Check sheet for the modelled part. Datum: model origin and axes. Units: mm. Face numbers are marked on the shaded views. A direction names the side the tool comes from. Give positions to 0.01 mm unless a question says otherwise; leave off trailing zeros. Order: outer loops, then holes, each group sorted by start corner. A loop starts at its lowest first (then second) coordinate and runs counter-clockwise, first axis right, second up.
Item 1: Sectioned sample at A-A on x = 0. Record the boundary of the cut face in (y, z), and give its area (3 significant figures).
Item 2: Sectioned sample at B-B on z = 0.7. Record the boundary of the cut face in (x, y) (3 decimals), and give its area (3 significant figures).
Item 3: Access from +Z, -Z, +X, -X, +Y, -Y to the whole of each face (thin tool, end or side, straight path). Record for the marked faces 1, 2 and 3.
Item 4: Release check for a two-part mould opening along X. For the marked faces 4, 5, 6 and 7 record: released by +X, released by -X, zero draft, split by the parting line, or undercut.
Item 5: Material ranges on line 1 along X through (y, z) = (-1, 2.4); line 2 along Y through (x, z) = (0, 0.75); line 3 along Z through (x, y) = (6.5, -9.5), recorded low to high.
Item 6: Gauge pin test, flat ends, axial feed: P1, Ø3.5, axis at x = -6.5, y = -9.5, coming from the +Z side; P2, Ø0.6, axis at x = -2.5, y = 5.5, coming from the +Z side; P3, Ø0.8, axis at x = -11.5, y = -0.5, coming from the +Z side. Record the tip position at first contact, or that the pin passes through.
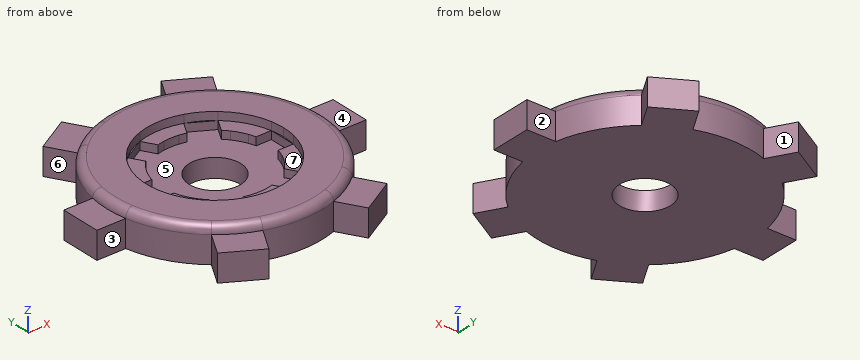
from build123d import *

# Parameters (mm, degrees)
F2_DEPTH = 2.54
F3_R     = 7.6884407039
F3_R_2   = 2.4226171542
F4_DEPTH = 1.778
F6_DEPTH = 0.762
F7_R     = 0.76199


# Not quite as in the source:
# - a fillet or chamfer is up to 0.001 mm smaller than in the source, because OpenCascade refuses the exact size


with BuildPart() as f2:
    # F1 (on Top) → F2 (new body)
    with BuildSketch(Plane.XY):
        with BuildLine():
            ThreePointArc((9.9798083649, -1.905), (10.1148517781, -0.9567515385), (10.16, 0))
            ThreePointArc((10.16, 0), (10.1148517781, 0.9567515385), (9.9798083649, 1.905))
            Line((9.9798083649, 1.905), (4.7092860393, 1.905))
            ThreePointArc((4.7092860393, 1.905), (4.8244462237, 1.5909489729), (4.9186888497, 1.27))
            Line((4.9186888497, 1.27), (6.35, 1.27))
            Line((6.35, 1.27), (6.35, -1.27))
            Line((6.35, -1.27), (4.9186888497, -1.27))
            ThreePointArc((4.9186888497, -1.27), (4.8244462237, -1.5909489729), (4.7092860393, -1.905))
            Line((4.7092860393, -1.905), (9.9798083649, -1.905))
        make_face()
        with BuildLine():
            ThreePointArc((9.9798083649, 1.905), (10.1148517781, 0.9567515385), (10.16, 0))
            ThreePointArc((10.16, 0), (10.1148517781, -0.9567515385), (9.9798083649, -1.905))
            Line((9.9798083649, -1.905), (12.7, -1.905))
            Line((12.7, -1.905), (12.7, 1.905))
            Line((12.7, 1.905), (9.9798083649, 1.905))
        make_face()
        with BuildLine():
            Line((4.7092860393, 1.905), (9.9798083649, 1.905))
            ThreePointArc((9.9798083649, 1.905), (8.7988181024, 5.08), (6.6396825767, 7.6902675689))
            Line((6.6396825767, 7.6902675689), (4.0044214139, 3.1258613437))
            ThreePointArc((4.0044214139, 3.1258613437), (4.3994090512, 2.54), (4.7092860393, 1.905))
        make_face()
        with BuildLine():
            ThreePointArc((6.6396825767, -7.6902675689), (8.7988181024, -5.08), (9.9798083649, -1.905))
            Line((9.9798083649, -1.905), (4.7092860393, -1.905))
            ThreePointArc((4.7092860393, -1.905), (4.3994090512, -2.54), (4.0044214139, -3.1258613437))
            Line((4.0044214139, -3.1258613437), (6.6396825767, -7.6902675689))
        make_face()
        with BuildLine():
            Line((4.0044214139, 3.1258613437), (6.6396825767, 7.6902675689))
            ThreePointArc((6.6396825767, 7.6902675689), (5.08, 8.7988181024), (3.3401257882, 9.5952675689))
            Line((3.3401257882, 9.5952675689), (0.7048646254, 5.0308613437))
            ThreePointArc((0.7048646254, 5.0308613437), (1.0344208852, 4.9735674754), (1.359492162, 4.8947094971))
            Line((1.359492162, 4.8947094971), (2.0751477372, 6.134261314))
            Line((2.0751477372, 6.134261314), (4.2748522628, 4.864261314))
            Line((4.2748522628, 4.864261314), (3.5591966876, 3.6247094971))
            ThreePointArc((3.5591966876, 3.6247094971), (3.7900253385, 3.3826185025), (4.0044214139, 3.1258613437))
        make_face()
        with BuildLine():
            ThreePointArc((3.3401257882, 9.5952675689), (5.08, 8.7988181024), (6.6396825767, 7.6902675689))
            Line((6.6396825767, 7.6902675689), (7.9997783942, 10.0460226281))
            Line((7.9997783942, 10.0460226281), (4.7002216058, 11.9510226281))
            Line((4.7002216058, 11.9510226281), (3.3401257882, 9.5952675689))
        make_face()
        with BuildLine():
            Line((7.9997783942, -10.0460226281), (6.6396825767, -7.6902675689))
            ThreePointArc((6.6396825767, -7.6902675689), (5.08, -8.7988181024), (3.3401257882, -9.5952675689))
            Line((3.3401257882, -9.5952675689), (4.7002216058, -11.9510226281))
            Line((4.7002216058, -11.9510226281), (7.9997783942, -10.0460226281))
        make_face()
        with BuildLine():
            ThreePointArc((3.3401257882, -9.5952675689), (5.08, -8.7988181024), (6.6396825767, -7.6902675689))
            Line((6.6396825767, -7.6902675689), (4.0044214139, -3.1258613437))
            ThreePointArc((4.0044214139, -3.1258613437), (3.7900253385, -3.3826185025), (3.5591966876, -3.6247094971))
            Line((3.5591966876, -3.6247094971), (4.2748522628, -4.864261314))
            Line((4.2748522628, -4.864261314), (2.0751477372, -6.134261314))
            Line((2.0751477372, -6.134261314), (1.359492162, -4.8947094971))
            ThreePointArc((1.359492162, -4.8947094971), (1.0344208852, -4.9735674754), (0.7048646254, -5.0308613437))
            Line((0.7048646254, -5.0308613437), (3.3401257882, -9.5952675689))
        make_face()
        with BuildLine():
            Line((0.7048646254, 5.0308613437), (3.3401257882, 9.5952675689))
            ThreePointArc((3.3401257882, 9.5952675689), (0, 10.16), (-3.3401257882, 9.5952675689))
            Line((-3.3401257882, 9.5952675689), (-0.7048646254, 5.0308613437))
            ThreePointArc((-0.7048646254, 5.0308613437), (0, 5.08), (0.7048646254, 5.0308613437))
        make_face()
        with BuildLine():
            ThreePointArc((-3.3401257882, -9.5952675689), (0, -10.16), (3.3401257882, -9.5952675689))
            Line((3.3401257882, -9.5952675689), (0.7048646254, -5.0308613437))
            ThreePointArc((0.7048646254, -5.0308613437), (0, -5.08), (-0.7048646254, -5.0308613437))
            Line((-0.7048646254, -5.0308613437), (-3.3401257882, -9.5952675689))
        make_face()
        with BuildLine():
            Line((-0.7048646254, 5.0308613437), (-3.3401257882, 9.5952675689))
            ThreePointArc((-3.3401257882, 9.5952675689), (-5.08, 8.7988181024), (-6.6396825767, 7.6902675689))
            Line((-6.6396825767, 7.6902675689), (-4.0044214139, 3.1258613437))
            ThreePointArc((-4.0044214139, 3.1258613437), (-3.7900253385, 3.3826185025), (-3.5591966876, 3.6247094971))
            Line((-3.5591966876, 3.6247094971), (-4.2748522628, 4.864261314))
            Line((-4.2748522628, 4.864261314), (-2.0751477372, 6.134261314))
            Line((-2.0751477372, 6.134261314), (-1.359492162, 4.8947094971))
            ThreePointArc((-1.359492162, 4.8947094971), (-1.0344208852, 4.9735674754), (-0.7048646254, 5.0308613437))
        make_face()
        with BuildLine():
            ThreePointArc((-6.6396825767, 7.6902675689), (-5.08, 8.7988181024), (-3.3401257882, 9.5952675689))
            Line((-3.3401257882, 9.5952675689), (-4.7002216058, 11.9510226281))
            Line((-4.7002216058, 11.9510226281), (-7.9997783942, 10.0460226281))
            Line((-7.9997783942, 10.0460226281), (-6.6396825767, 7.6902675689))
        make_face()
        with BuildLine():
            Line((-4.7002216058, -11.9510226281), (-3.3401257882, -9.5952675689))
            ThreePointArc((-3.3401257882, -9.5952675689), (-5.08, -8.7988181024), (-6.6396825767, -7.6902675689))
            Line((-6.6396825767, -7.6902675689), (-7.9997783942, -10.0460226281))
            Line((-7.9997783942, -10.0460226281), (-4.7002216058, -11.9510226281))
        make_face()
        with BuildLine():
            ThreePointArc((-6.6396825767, -7.6902675689), (-5.08, -8.7988181024), (-3.3401257882, -9.5952675689))
            Line((-3.3401257882, -9.5952675689), (-0.7048646254, -5.0308613437))
            ThreePointArc((-0.7048646254, -5.0308613437), (-1.0344208852, -4.9735674754), (-1.359492162, -4.8947094971))
            Line((-1.359492162, -4.8947094971), (-2.0751477372, -6.134261314))
            Line((-2.0751477372, -6.134261314), (-4.2748522628, -4.864261314))
            Line((-4.2748522628, -4.864261314), (-3.5591966876, -3.6247094971))
            ThreePointArc((-3.5591966876, -3.6247094971), (-3.7900253385, -3.3826185025), (-4.0044214139, -3.1258613437))
            Line((-4.0044214139, -3.1258613437), (-6.6396825767, -7.6902675689))
        make_face()
        with BuildLine():
            Line((-4.0044214139, 3.1258613437), (-6.6396825767, 7.6902675689))
            ThreePointArc((-6.6396825767, 7.6902675689), (-8.7988181024, 5.08), (-9.9798083649, 1.905))
            Line((-9.9798083649, 1.905), (-4.7092860393, 1.905))
            ThreePointArc((-4.7092860393, 1.905), (-4.3994090512, 2.54), (-4.0044214139, 3.1258613437))
        make_face()
        with BuildLine():
            ThreePointArc((-9.9798083649, -1.905), (-8.7988181024, -5.08), (-6.6396825767, -7.6902675689))
            Line((-6.6396825767, -7.6902675689), (-4.0044214139, -3.1258613437))
            ThreePointArc((-4.0044214139, -3.1258613437), (-4.3994090512, -2.54), (-4.7092860393, -1.905))
            Line((-4.7092860393, -1.905), (-9.9798083649, -1.905))
        make_face()
        with BuildLine():
            Line((-4.7092860393, 1.905), (-9.9798083649, 1.905))
            ThreePointArc((-9.9798083649, 1.905), (-10.16, 0), (-9.9798083649, -1.905))
            Line((-9.9798083649, -1.905), (-4.7092860393, -1.905))
            ThreePointArc((-4.7092860393, -1.905), (-4.8244462237, -1.5909489729), (-4.9186888497, -1.27))
            Line((-4.9186888497, -1.27), (-6.35, -1.27))
            Line((-6.35, -1.27), (-6.35, 1.27))
            Line((-6.35, 1.27), (-4.9186888497, 1.27))
            ThreePointArc((-4.9186888497, 1.27), (-4.8244462237, 1.5909489729), (-4.7092860393, 1.905))
        make_face()
        with BuildLine():
            ThreePointArc((-9.9798083649, -1.905), (-10.16, 0), (-9.9798083649, 1.905))
            Line((-9.9798083649, 1.905), (-12.7, 1.905))
            Line((-12.7, 1.905), (-12.7, -1.905))
            Line((-12.7, -1.905), (-9.9798083649, -1.905))
        make_face()
    extrude(amount=F2_DEPTH)

    # F3 (on face) → F4 (join)
    with BuildSketch(Plane.XY):
        Circle(F3_R)
        Circle(F3_R_2, mode=Mode.SUBTRACT)
    extrude(amount=F4_DEPTH)

    # F5 (on face) → F6 (join)
    with BuildSketch(Plane.XY.offset(2.54)):
        with BuildLine():
            ThreePointArc((9.9798083649, -1.905), (10.1148517781, -0.9567515385), (10.16, 0))
            ThreePointArc((10.16, 0), (10.1148517781, 0.9567515385), (9.9798083649, 1.905))
            ThreePointArc((9.9798083649, 1.905), (8.7988181024, 5.08), (6.6396825767, 7.6902675689))
            ThreePointArc((6.6396825767, 7.6902675689), (5.08, 8.7988181024), (3.3401257882, 9.5952675689))
            ThreePointArc((3.3401257882, 9.5952675689), (0, 10.16), (-3.3401257882, 9.5952675689))
            ThreePointArc((-3.3401257882, 9.5952675689), (-5.08, 8.7988181024), (-6.6396825767, 7.6902675689))
            ThreePointArc((-6.6396825767, 7.6902675689), (-8.7988181024, 5.08), (-9.9798083649, 1.905))
            ThreePointArc((-9.9798083649, 1.905), (-10.16, 0), (-9.9798083649, -1.905))
            ThreePointArc((-9.9798083649, -1.905), (-8.7988181024, -5.08), (-6.6396825767, -7.6902675689))
            ThreePointArc((-6.6396825767, -7.6902675689), (-5.08, -8.7988181024), (-3.3401257882, -9.5952675689))
            ThreePointArc((-3.3401257882, -9.5952675689), (0, -10.16), (3.3401257882, -9.5952675689))
            ThreePointArc((3.3401257882, -9.5952675689), (5.08, -8.7988181024), (6.6396825767, -7.6902675689))
            ThreePointArc((6.6396825767, -7.6902675689), (8.7988181024, -5.08), (9.9798083649, -1.905))
        make_face()
        with BuildLine():
            ThreePointArc((6.35, 1.27), (6.4442393992, 0.6381054508), (6.4757547823, 0))
            ThreePointArc((6.4757547823, 0), (6.4442393992, -0.6381054508), (6.35, -1.27))
            ThreePointArc((6.35, -1.27), (5.6081681501, -3.2378773911), (4.2748522628, -4.864261314))
            ThreePointArc((4.2748522628, -4.864261314), (3.2378773911, -5.6081681501), (2.0751477372, -6.134261314))
            ThreePointArc((2.0751477372, -6.134261314), (0, -6.4757547823), (-2.0751477372, -6.134261314))
            ThreePointArc((-2.0751477372, -6.134261314), (-3.2378773911, -5.6081681501), (-4.2748522628, -4.864261314))
            ThreePointArc((-4.2748522628, -4.864261314), (-5.6081681501, -3.2378773911), (-6.35, -1.27))
            ThreePointArc((-6.35, -1.27), (-6.4757547823, 0), (-6.35, 1.27))
            ThreePointArc((-6.35, 1.27), (-5.6081681501, 3.2378773911), (-4.2748522628, 4.864261314))
            ThreePointArc((-4.2748522628, 4.864261314), (-3.2378773911, 5.6081681501), (-2.0751477372, 6.134261314))
            ThreePointArc((-2.0751477372, 6.134261314), (0, 6.4757547823), (2.0751477372, 6.134261314))
            ThreePointArc((2.0751477372, 6.134261314), (3.2378773911, 5.6081681501), (4.2748522628, 4.864261314))
            ThreePointArc((4.2748522628, 4.864261314), (5.6081681501, 3.2378773911), (6.35, 1.27))
        make_face(mode=Mode.SUBTRACT)
    extrude(amount=F6_DEPTH)

    # F7 (radius 0.762 in the source; OpenCascade refuses exactly that, so slightly less here)
    f7_edges = [f2.edges().sort_by_distance(p)[0] for p in [
        (9.979808, 1.905, 3.302),
    ]]
    fillet(f7_edges, radius=F7_R)


solid = f2.part
Report:
1. outline: (-10.16, 0) - (-2.42, 0) - (-2.42, 1.78) - (-5.08, 1.78) - (-5.08, 2.54) - (-6.48, 2.54) - (-6.48, 3.3) - (-9.4, 3.3) arc R0.76 ccw to (-10.16, 2.54) - close; (2.42, 0) - (10.16, 0) - (10.16, 2.54) arc R0.76 ccw to (9.4, 3.3) - (6.48, 3.3) - (6.48, 2.54) - (5.08, 2.54) - (5.08, 1.78) - (2.42, 1.78) - close
1. area: 40.6 mm2
2. outline: (-12.7, -1.905) - (-9.98, -1.905) arc R10.16 ccw to (-6.64, -7.69) - (-8, -10.046) - (-4.7, -11.951) - (-3.34, -9.595) arc R10.16 ccw to (3.34, -9.595) - (4.7, -11.951) - (8, -10.046) - (6.64, -7.69) arc R10.16 ccw to (9.98, -1.905) - (12.7, -1.905) - (12.7, 1.905) - (9.98, 1.905) arc R10.16 ccw to (6.64, 7.69) - (8, 10.046) - (4.7, 11.951) - (3.34, 9.595) arc R10.16 ccw to (-3.34, 9.595) - (-4.7, 11.951) - (-8, 10.046) - (-6.64, 7.69) arc R10.16 ccw to (-9.98, 1.905) - (-12.7, 1.905) - close; hole circle Ø4.845 at (0, 0)
2. area: 365 mm2
3. face 1: +Z, -Z, +Y
3. face 2: +Z, -Z, +X, +Y
3. face 3: +Z, -Z, -X, -Y
4. face 4: zero draft
4. face 5: undercut
4. face 6: released by -X
4. face 7: undercut
5. line 1: x = -12.7 to -6.35, 6.35 to 12.7
5. line 2: y = -10.16 to -2.42, 2.42 to 10.16
5. line 3: z = 0 to 2.54
6. P1: stops at z = 3.21
6. P2: stops at z = 1.78
6. P3: stops at z = 2.54
